from build123d import *

# Parameters (mm, degrees)
F0_R     = 50.8
F1_DEPTH = 19.05
F2_SIZE  = 12.7
F4_D     = 12.7
F5_D     = 15.875


# Not quite as in the source:
# - a length typed as a fraction of an inch, garbled in the dataset ("3 / 203.2 mm" for 3/8 in), is restored


with BuildPart() as f1:
    # F0 (on Top) → F1 (new body, symmetric)
    with BuildSketch(Plane.XY):
        Circle(F0_R)
    extrude(amount=F1_DEPTH, both=True)

    # F2
    f2_edges = [f1.edges().sort_by_distance(p)[0] for p in [
        (-50.8, 0, 19.05),
    ]]
    chamfer(f2_edges, length=F2_SIZE)

    # F4 (through all)
    with Locations(Plane(origin=(0, 0, -19.05), x_dir=(1, 0, 0), z_dir=(0, 0, -1))):
        with Locations((-22.4506403027, 22.4506403027), (-22.4506403027, -22.4506403027), (22.4506403027, -22.4506403027), (22.4506403027, 22.4506403027)):
            Hole(F4_D / 2)

    # F5 (through all)
    with Locations(Plane(origin=(0, 0, -19.05), x_dir=(1, 0, 0), z_dir=(0, 0, -1))):
        with Locations((0, 0)):
            Hole(F5_D / 2)


solid = f1.part
The listing builds one solid part. Answer for the finished solid, in the listing's coordinates (mm). Coordinates: 2 decimals unless noted, no trailing zeros. Order: outer loops, then holes, each group sorted by start corner. A loop starts at its lowest first (then second) coordinate and runs counter-clockwise, first axis right, second up.
Q1. Consider line 1 (X direction, y = -17.5, z = -10); line 2 (Y direction, x = -17, z = -13); line 3 (Y direction, x = 0, z = 1). Determine where each line is inside the solid, lowest interval first.
Q2. For a pull along Y with two mould halves and no side action, classify faces 1 (the face through (-11.012, -49.592, -6.172)), 2 (the face through (8, -8, 19.05)), 3 (the face through (1.72, 7.75, 0.27)) as pulls with the +Y half, pulls with the -Y half, needs draft (parallel to the pull), parting line crosses it, or undercut.
Q3. A cutting plane is placed at A-A, the plane x = 0. Write down the section's boundary in (y, z).
Q4. Given P1, Ø1.5, axis at y = -20.5, z = 14, coming from the -X side; P2, Ø11.5, axis at x = -22.45, y = 22.45, coming from the +Z side; P3, Ø5, axis at x = -35, y = -37, coming from the +Z side; P4, Ø1, axis at x = -38, y = 25, coming from the +Z side, each flat-ended and moving along its own axis, determine where each tip first touches the part or whether it passes through.
Q5. A cutting plane is placed at C-C, the plane z = 13. State how many separate pieces and enclosed holes the cut face has, and give its area (3 significant figures).
Answers follow:
1. line 1: x = -47.69 to -26.43, -18.47 to 18.47, 26.43 to 47.69
1. line 2: y = -47.87 to -25.71, -19.19 to 19.19, 25.71 to 47.87
1. line 3: y = -50.8 to -7.94, 7.94 to 50.8
2. face 1: parting line crosses it
2. face 2: needs draft
2. face 3: undercut
3. outline: (-50.8, -19.05) - (-7.94, -19.05) - (-7.94, 19.05) - (-38.1, 19.05) - (-50.8, 6.35) - close; (7.94, -19.05) - (50.8, -19.05) - (50.8, 6.35) - (38.1, 19.05) - (7.94, 19.05) - close
4. P1: stops at x = -38.91
4. P2: passes through
4. P3: stops at z = 8.72
4. P4: stops at z = 12.16
5. separate pieces: 1
5. enclosed holes: 5
5. area: 5,420 mm2
